The model under review builds one solid part; all positions refer to its coordinate system, in mm. A direction names the side the tool comes from. Coordinates: 2 decimals unless noted, no trailing zeros. Write each loop counter-clockwise with the first axis right and the second up, starting at its lowest first coordinate (ties: lowest second). Pieces come first, ordered by that corner, then holes. Notation, with made-up numbers: (8, 55.25) - (60, 55.25) arc R21 ccw to (60, 92.25) - close; hole circle Ø11 at (-2, -12). An arc over 180 degrees is marked (long way). Return JSON: item names as keys, results as strings. Group by question number.
(1) Draft analysis for pull direction X (two halves, no side actions). For faces 4 (the face through (51, 33, -23)), 5 (the face through (33, 12, -16)), 6 (the face through (-41, 9, -32)), 7 (the face through (13, 33, -23)), state which applies: released by +X, released by -X, zero draft, split by the parting line, or undercut.
(2) For pin 1 Ø13 at (y, z) = (27.5, -28.5) entering from -X; pin 2 Ø8 at (x, z) = (-25.5, -36) entering from +Y; pin 3 Ø5 at (x, y) = (31.5, 22.5) entering from +Z, all flat-tipped, find the tip position at first contact; note any pin that passes through.
(3) We need section D-D on y = 24. State the section outline as (x, z) points.
(4) We need section C-C on z = -19. State the section outline as (x, y) points, then the cut area to 3 significant figures.
(5) Tool access review of faces 1 (the face through (64, 32, -32)), 2 (the face through (0, 32, -32)), 3 (the face through (32.27, 29.22, -25.63)): name each direction out of +Z, -Z, +X, -X, +Y, -Y from which nothing blocks a thin tool from reaching the whole face with its end or side.
(6) We need section B-B on z = -29.5. State the section outline as (x, y) points, then the cut area to 3 significant figures.
(7) We need section A-A on x = -16. State the section outline as (y, z) points.
(8) To check wall thickness, follow L1, parallel to X at y = 13.5, z = -32; L2, parallel to X at y = 13.5, z = -35; L3, parallel to X at y = 26, z = -20. State the ranges of each line that lie inside material, in increasing order. Write a range as from..to.
```python
from build123d import *

# Parameters (mm, degrees)
SKETCH2_W           = 64
SKETCH2_H           = 64
BOSS_EXTRUDE1_DEPTH = 45
SKETCH3_R           = 11
BOSS_EXTRUDE2_DEPTH = 19
SKETCH7_W           = 16
SKETCH7_H           = 45
CUT_EXTRUDE2_DEPTH  = 148
SKETCH9_W           = 64
SKETCH9_H           = 16
CUT_EXTRUDE4_DEPTH  = 148
SKETCH10_W          = 38
SKETCH10_H          = 19
CUT_EXTRUDE5_DEPTH  = 32
BOSS_EXTRUDE4_DEPTH = 42


with BuildPart() as part:
    # Sketch2 → Boss-Extrude1 (new body)
    with BuildSketch(Plane(origin=(0, 0, 0), x_dir=(1, 0, 0), z_dir=(0, 1, 0))):
        with Locations((32, 32)):
            Rectangle(SKETCH2_W, SKETCH2_H)
    extrude(amount=BOSS_EXTRUDE1_DEPTH)

    # Sketch3 → Boss-Extrude2 (add)
    # profile 1 of 2: a face of its own
    with BuildSketch(Plane(origin=(0, 0, 0), x_dir=(1, 0, 0), z_dir=(0, 1, 0))):
        with BuildLine():
            Line((-25, 48), (0, 48))
            Line((0, 48), (0, 16))
            Line((0, 16), (-25, 16))
            ThreePointArc((-25, 16), (-41, 32), (-25, 48))
        make_face()
        with Locations(Location((-25, 32, 0), (0, 0, 270))):
            Circle(SKETCH3_R, mode=Mode.SUBTRACT)
    # profile 2 of 2: a face of its own
    with BuildSketch(Plane(origin=(0, 0, 0), x_dir=(1, 0, 0), z_dir=(0, 1, 0))):
        with BuildLine():
            Line((89, 48), (64, 48))
            Line((64, 48), (64, 16))
            Line((64, 16), (89, 16))
            ThreePointArc((89, 16), (105, 32), (89, 48))
        make_face()
        with Locations(Location((89, 32, 0), (0, 0, 270))):
            Circle(SKETCH3_R, mode=Mode.SUBTRACT)
    extrude(amount=BOSS_EXTRUDE2_DEPTH)

    # Sketch7 → Cut-Extrude2 (cut)
    with BuildSketch(Plane.ZY):
        with Locations((-8, 22.5)):
            Rectangle(SKETCH7_W, SKETCH7_H)
    extrude(amount=-CUT_EXTRUDE2_DEPTH, mode=Mode.SUBTRACT)

    # Sketch9 → Cut-Extrude4 (cut)
    with BuildSketch(Plane(origin=(0, 45, 0), x_dir=(1, 0, 0), z_dir=(0, 1, 0))):
        with Locations((32, 56)):
            Rectangle(SKETCH9_W, SKETCH9_H)
    extrude(amount=-CUT_EXTRUDE4_DEPTH, mode=Mode.SUBTRACT)

    # Sketch10 → Cut-Extrude5 (cut)
    with BuildSketch(Plane(origin=(0, 45, 0), x_dir=(1, 0, 0), z_dir=(0, 1, 0))):
        with Locations((32, 25.5)):
            Rectangle(SKETCH10_W, SKETCH10_H)
    extrude(amount=-CUT_EXTRUDE5_DEPTH, mode=Mode.SUBTRACT)

    # Sketch12 → Boss-Extrude4 (add)
    with BuildSketch(Plane.ZY.offset(-51)):
        Polygon((-35, 45), (-16, 13), (-35, 13), align=None)
    extrude(amount=BOSS_EXTRUDE4_DEPTH)


solid = part.part
```
Ans:
{
 "1": {"face 4": "undercut", "face 5": "zero draft", "face 6": "released by -X", "face 7": "undercut"},
 "2": {"pin 1": "x = 0", "pin 2": "through", "pin 3": "z = -20.16"},
 "3": {"outline": "(0, -48) - (64, -48) - (64, -16) - (51, -16) - (51, -22.53) - (13, -22.53) - (13, -16) - (0, -16) - close"},
 "4": {"outline": "(-34.33, 0) - (98.33, 0) - (98.33, 19) - (64, 19) - (64, 45) - (51, 45) - (51, 18.05) - (13, 18.05) - (13, 45) - (0, 45) - (0, 19) - (-34.33, 19) - close", "area": "3,160 mm²"},
 "5": {"face 1": "+Z, -Z, +X, +Y", "face 2": "+Z, -Z, -X, +Y", "face 3": "+Z, +Y"},
 "6": {"outline": "(-40.8, 0) - (-35.71, 0) - (-35.71, 19) - (-40.8, 19) - close; (-14.29, 0) - (78.29, 0) - (78.29, 19) - (64, 19) - (64, 45) - (51, 45) - (51, 35.74) - (13, 35.74) - (13, 45) - (0, 45) - (0, 19) - (-14.29, 19) - close; (99.71, 0) - (104.8, 0) - (104.8, 19) - (99.71, 19) - close", "area": "3,260 mm²"},
 "7": {"outline": "(0, -48) - (19, -48) - (19, -38.32) - (0, -38.32) - close; (0, -25.68) - (19, -25.68) - (19, -16) - (0, -16) - close"},
 "8": {"L1": "-41..-36, -14..78, 100..105", "L2": "-40.72..-35.58, -14.42..78.42, 99.58..104.72", "L3": "0..13, 51..64"}
}
